CAD build for the part. Positions are in the model's coordinates, mm. Face numbers are marked on the shaded views. A direction names the side the tool comes from. Give positions to 0.01 mm unless a question says otherwise; leave off trailing zeros. Loops run counter-clockwise (first coordinate to the right, second up) from the corner with the lowest first, then second, coordinate; pieces in that order, holes last. Notation, with made-up numbers: M 38.5,9 L 57.5,9 A14 ccw 57.5,15 Z; hole C 41.5,51.5 d8. An arc over 180 degrees is marked long. Answer as CSV lines item,"result".
Autodesk Inventor part; units mm, degrees
ref_plane "YZ Plane" through (0, 0, 0) normal (1, 0, 0) x (0, 1, 0)
ref_plane "XZ Plane" through (0, 0, 0) normal (0, 1, 0) x (-1, 0, 0)
ref_plane "XY Plane" through (0, 0, 0) normal (0, 0, 1) x (1, 0, 0)
sketch "Sketch1" plane through (0, 0, 0) normal (0, 0, 1) x (1, 0, 0)
  line L0 (0, 0) -> (28, 0)
  line L1 (28, 0) -> (28, -53.6)
  line L2 (28, -53.6) -> (0, -53.6)
  line L3 (0, -53.6) -> (0, 0)
  dimension "d0" = 28
  dimension "d1" = 53.6
extrude "Extrusion1" add sketch "Sketch1" along normal blind 32.4
sketch "Sketch2" plane through (0, 0, 32.4) normal (0, 0, 1) x (1, 0, 0)
  circle A0 centre (14, -11) radius 11
  dimension "d5" = 22
extrude "Extrusion2" add sketch "Sketch2" along normal blind 4.54
sketch "Sketch3" plane through (0, 0, 0) normal (0, 0, -1) x (-1, 0, 0)
  line L0 (0, 0) -> (-28, 0)
  line L1 (0, 0) -> (-14, 0)
  line L2 (-14, 0) -> (-14, -11)
  circle A0 centre (-14, -11) radius 5
  dimension "d8" = 14
  dimension "d9" = 11
  dimension "d10" = 10
extrude "Extrusion3" add sketch "Sketch3" along normal blind 2.4
sketch "Sketch4" plane through (0, -53.6, 0) normal (0, -1, 0) x (1, 0, 0)
  line L0 (0, 0) -> (28, 0)
  line L1 (0, 0) -> (0, 32.4)
  line L2 (6.5, 23.7) -> (6.5, 8.7)
  line L3 (6.5, 8.7) -> (21.5, 8.7)
  line L4 (21.5, 8.7) -> (21.5, 23.7)
  circle A0 centre (6.5, 23.7) radius 1.45
  circle A1 centre (6.5, 8.7) radius 1.45
  circle A2 centre (21.5, 8.7) radius 1.45
  circle A3 centre (21.5, 23.7) radius 1.45
  dimension "d17" = 15
  dimension "d18" = 15
  dimension "d19" = 2.9
  dimension "d20" = 2.9
  dimension "d21" = 2.9
  dimension "d22" = 2.9
extrude "Extrusion4" add sketch "Sketch4" along normal blind 1
properties part number "ax_18_replace"
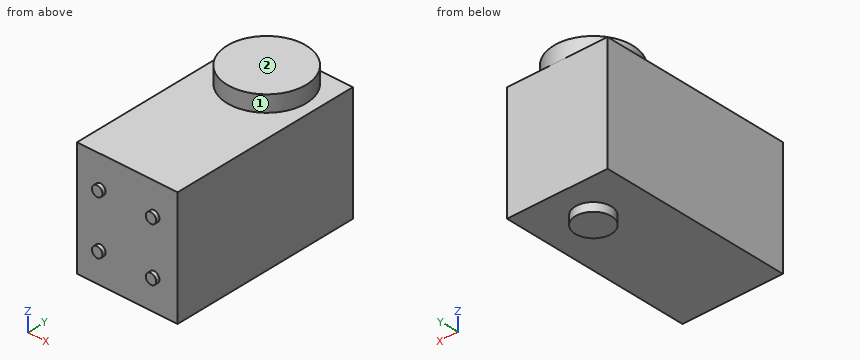
1) Which spindle directions (+Z, -Z, +X, -X, +Y, -Y) get a long thin tool onto all of the face, cutting with end or side? Do the marked faces 1 and 2. Say none if no direction does.
Answer below:
face 1,"+Z"
face 2,"+Z, +X, -X, +Y, -Y"
2) Band-saw the part on D-D on y = -18.5. Give the cut face in (x, z).
Answer below:
outline,"M 0,0 L 28,0 L 28,32.4 L 22.05,32.4 L 22.05,36.94 L 5.95,36.94 L 5.95,32.4 L 0,32.4 Z"
3) Band-saw the part on C-C on z = 20. Give the cut face in (x, y).
Answer below:
outline,"M 0,-53.6 L 28,-53.6 L 28,0 L 0,0 Z"
4) Band-saw the part on A-A on y = -11. Give the cut face in (x, z).
Answer below:
outline,"M 0,0 L 9,0 L 9,-2.4 L 19,-2.4 L 19,0 L 28,0 L 28,32.4 L 25,32.4 L 25,36.94 L 3,36.94 L 3,32.4 L 0,32.4 Z"
5) Band-saw the part on B-B on x = 21.5. Give the cut face in (y, z), and give its area (3 significant figures).
Answer below:
outline,"M -54.6,7.25 L -53.6,7.25 L -53.6,0 L 0,0 L 0,32.4 L -2.95,32.4 L -2.95,36.94 L -19.05,36.94 L -19.05,32.4 L -53.6,32.4 L -53.6,25.15 L -54.6,25.15 L -54.6,22.25 L -53.6,22.25 L -53.6,10.15 L -54.6,10.15 Z"
area,"1,820 mm^2"
6) Drill centre lines: line 1 (Z direction, x = 8, y = -35); line 2 (Z direction, x = 5, y = -16); line 3 (Y direction, x = 5.5, z = 31). Where is each one in solid material? Low to high. Write a range as from..to.
Answer below:
line 1,"z = 0..32.4"
line 2,"z = 0..36.94"
line 3,"y = -53.6..0"
